from build123d import *

# Parameters (mm, degrees)
SKETCH_1_W           = 4.2
SKETCH_1_H           = 3.2
EXTRUDE_1_DEPTH      = 5
SKETCH_2_W           = 3.6
SKETCH_2_H           = 2.6
CUT_EXTRUDE_2_DEPTH  = 4.5
SKETCH_10_W          = 1.719860591
SKETCH_10_H          = 0.3
CUT_EXTRUDE_6_DEPTH  = 1.5
SKETCH_12_W          = 0.497980778
SKETCH_12_H          = 0.499968878
SKETCH_12_W_2        = 0.49954636
EXTRUDE_2_DEPTH      = 4
EXTRUDE_2_DEPTH_BACK = 2
CHAMFER_2_SIZE       = 0.1
CHAMFER_3_SIZE       = 0.1


with BuildPart() as part:
    # 草图1 → 凸台-拉伸1 (new body)
    with BuildSketch(Plane.XY):
        Rectangle(SKETCH_1_W, SKETCH_1_H)
    extrude(amount=EXTRUDE_1_DEPTH)

    # 草图2 → 切除-拉伸2 (cut)
    with BuildSketch(Plane.XY.offset(5)):
        Rectangle(SKETCH_2_W, SKETCH_2_H)
    extrude(amount=-CUT_EXTRUDE_2_DEPTH, mode=Mode.SUBTRACT)

    # 草图10 → 切除-拉伸6 (cut)
    with BuildSketch(Plane.XY.offset(5)):
        with Locations((-0.021149262, 1.45)):
            Rectangle(SKETCH_10_W, SKETCH_10_H)
    extrude(amount=-CUT_EXTRUDE_6_DEPTH, mode=Mode.SUBTRACT)

    # 草图12 → 凸台-拉伸2 (add, two sides)
    with BuildSketch(Plane.XY.offset(0.5)) as extrude_2_sk:
        with Locations((-0.7, -0.4)):
            Rectangle(SKETCH_12_W, SKETCH_12_H)
        with Locations((0.7, -0.4)):
            Rectangle(SKETCH_12_W_2, SKETCH_12_H)
    extrude(amount=EXTRUDE_2_DEPTH)
    extrude(extrude_2_sk.sketch, amount=-EXTRUDE_2_DEPTH_BACK)

    # 倒角2
    chamfer_2_edges = [part.edges().sort_by_distance(p)[0] for p in [
        (-0.451009611, -0.4, 4.5),
        (-0.7, -0.150015561, 4.5),
        (-0.948990389, -0.4, 4.5),
        (-0.7, -0.649984439, 4.5),
        (0.94977318, -0.4, 4.5),
        (0.7, -0.150015561, 4.5),
        (0.45022682, -0.4, 4.5),
        (0.7, -0.649984439, 4.5),
    ]]
    chamfer(chamfer_2_edges, length=CHAMFER_2_SIZE)

    # 倒角3
    chamfer_3_edges = [part.edges().sort_by_distance(p)[0] for p in [
        (-0.451009611, -0.4, -1.5),
        (-0.7, -0.649984439, -1.5),
        (-0.948990389, -0.4, -1.5),
        (-0.7, -0.150015561, -1.5),
        (0.94977318, -0.4, -1.5),
        (0.7, -0.649984439, -1.5),
        (0.45022682, -0.4, -1.5),
        (0.7, -0.150015561, -1.5),
    ]]
    chamfer(chamfer_3_edges, length=CHAMFER_3_SIZE)


solid = part.part
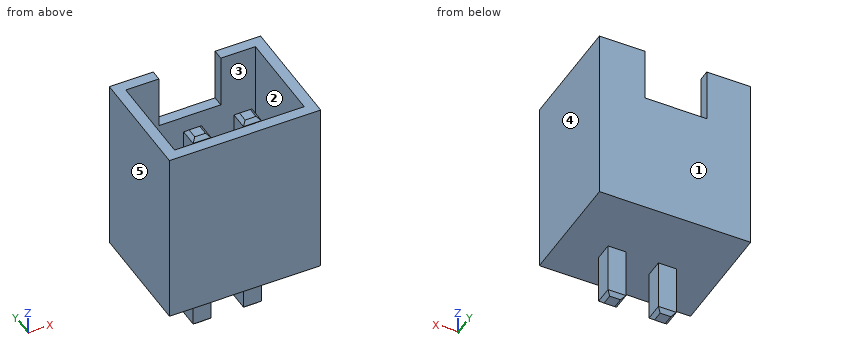
Design review of the part built by this model. Coordinates are the model's own, in mm. Face numbers are marked on the shaded views. A direction names the side the tool comes from. Give positions to 0.01 mm unless a question says otherwise; leave off trailing zeros. Loops run counter-clockwise (first coordinate to the right, second up) from the corner with the lowest first, then second, coordinate; pieces in that order, holes last. Notation, with made-up numbers: (44.25, 47) - (79.25, 47) arc R25 cw to (79.25, 80) - close; hole circle Ø8 at (29, -39.75). An arc over 180 degrees is marked (long way). Use CSV: the item, a comma, the result in double quotes. Start each with the question number.
1. Add section D-D (y = 0.2). State the section outline as (x, z) points, plus the area to 3 significant figures.
2. Machinability: for the marked faces 1 and 2, which of the approach directions +Z, -Z, +X, -X, +Y, -Y give a long, thin tool a straight path to every point of the face, cutting with its end or side? Answer none if there is none.
3. Wall thickness on L1, parallel to Y at x = -0.7, z = 2.75; L2, parallel to X at y = -0.3, z = 3; L3, parallel to Y at x = 1.15, z = 1.5: over which ranges is each line inside the solid? List them lowest first.
4. Add section C-C (x = 0.7). State the section outline as (y, z) points, plus the area to 3 significant figures.
5. Add section B-B (z = -0.25). State the section outline as (x, y) points.
6. Add section A-A (z = 0.75). State the section outline as (x, y) points.
7. Draft analysis for pull direction X (two halves, no side actions). For the marked faces 3, 4 and 5, state which applies: released by +X, released by -X, zero draft, split by the parting line, or undercut.
8. Insertion check: P1, Ø0.5, axis at y = -0.5, z = -0.5, coming from the -X side; P2, Ø1.3, axis at x = 0.5, y = -0.5, coming from the +Z side. Each pin has a flat end and moves straight along its axis. Give the tip position at first contact, or say it passes through.
Results found:
1,outline,"(-2.1, 0) - (2.1, 0) - (2.1, 5) - (1.8, 5) - (1.8, 0.5) - (-1.8, 0.5) - (-1.8, 5) - (-2.1, 5) - close"
1,area,"4.80 mm²"
2,face 1,"+Z, -Z, +X, -X, +Y"
2,face 2,"+Z"
3,L1,"y = -1.6 to -1.3, -0.65 to -0.15, 1.3 to 1.6"
3,L2,"x = -2.1 to -1.8, -0.95 to -0.45, 0.45 to 0.95, 1.8 to 2.1"
3,L3,"y = -1.6 to -1.3, 1.3 to 1.6"
4,outline,"(-1.6, 0) - (-0.65, 0) - (-0.65, -1.4) - (-0.55, -1.5) - (-0.25, -1.5) - (-0.15, -1.4) - (-0.15, 0) - (1.6, 0) - (1.6, 3.5) - (1.3, 3.5) - (1.3, 0.5) - (-0.15, 0.5) - (-0.15, 4.4) - (-0.25, 4.5) - (-0.55, 4.5) - (-0.65, 4.4) - (-0.65, 0.5) - (-1.3, 0.5) - (-1.3, 5) - (-1.6, 5) - close"
4,area,"6.58 mm²"
5,outline,"(-0.95, -0.65) - (-0.45, -0.65) - (-0.45, -0.15) - (-0.95, -0.15) - close; (0.45, -0.65) - (0.95, -0.65) - (0.95, -0.15) - (0.45, -0.15) - close"
6,outline,"(-2.1, -1.6) - (2.1, -1.6) - (2.1, 1.6) - (-2.1, 1.6) - close; (-0.95, -0.65) - (-0.45, -0.65) - (-0.45, -0.15) - (-0.95, -0.15) - close; (0.45, -0.65) - (0.95, -0.65) - (0.95, -0.15) - (0.45, -0.15) - close; hole (-1.8, -1.3) - (1.8, -1.3) - (1.8, 1.3) - (-1.8, 1.3) - close"
7,face 3,"undercut"
7,face 4,"released by +X"
7,face 5,"released by -X"
8,P1,"stops at x = -0.95"
8,P2,"stops at z = 4.5"
